Check sheet for the modelled part. Datum: model origin and axes. Units: mm. Face numbers are marked on the shaded views. A direction names the side the tool comes from. Round coordinates to 2 decimals unless told otherwise and drop trailing zeros. Write each loop counter-clockwise with the first axis right and the second up, starting at its lowest first coordinate (ties: lowest second). Pieces come first, ordered by that corner, then holes. Notation, with made-up numbers: (6.25, -26.5) -> (25.25, -26.5) arc R35 ccw to (25.25, 10.5) -> close; hole circle Ø1 at (25.25, -3). An arc over 180 degrees is marked (long way). One line per item, written item: value.
Autodesk Inventor part; units mm, degrees
ref_plane "YZ Plane" through (0, 0, 0) normal (1, 0, 0) x (0, 1, 0)
ref_plane "XZ Plane" through (0, 0, 0) normal (0, 1, 0) x (-1, 0, 0)
ref_plane "XY Plane" through (0, 0, 0) normal (0, 0, 1) x (1, 0, 0)
sketch "Sketch1" plane through (0, 0, 0) normal (0, 0, 1) x (1, 0, 0)
  line L0 (0, 0) -> (55, 0)
  line L1 (55, 0) -> (55, 80)
  line L2 (55, 80) -> (0, 80)
  line L3 (0, 80) -> (0, 0)
  dimension "d0" = 55
  dimension "d1" = 80
extrude "Base" add sketch "Sketch1" along normal blind 2
sketch "Sketch2" plane through (0, 0, 2) normal (0, 0, 1) x (1, 0, 0)
  line L0 (55, 0) -> (55, 80)
  line L1 (0, 80) -> (0, 0)
  line L2 (-2, 0) -> (57, 0)
  line L3 (57, 0) -> (57, 3)
  line L4 (57, 3) -> (-2, 3)
  line L5 (-2, 3) -> (-2, 0)
  dimension "d4" = 3
  dimension "d5" = 2
  dimension "d6" = 2
extrude "Back" add sketch "Sketch2" along normal blind 36.5 and the other way blind 2
sketch "Sketch6" plane through (0, 0, 2) normal (0, 0, 1) x (1, 0, 0)
  line L0 (0, 80) -> (0, 3)
  line L1 (0, 3) -> (55, 3)
  line L2 (55, 3) -> (55, 80)
  line L3 (2, 3) -> (53, 3)
  line L4 (53, 3) -> (53, 38)
  line L5 (53, 38) -> (2, 38)
  line L6 (2, 38) -> (2, 3)
  point P0 (0, 0)
  dimension "d29" = 35
  dimension "d30" = 2
  dimension "d31" = 2
extrude "Box" add sketch "Sketch6" along normal blind 13.5
chamfer "Chamfer3" distance 0.5 angle 45 8 edges at (0, 41.5, 0) (27.5, 80, 0) (55, 41.5, 0) (-1, 3, 0) (-2, 1.5, 0) (27.5, 0, 0) (57, 1.5, 0) (56, 3, 0)
chamfer "Chamfer4" distance 0.5 angle 45 3 edges at (-2, 0, 19.5) (27.5, 0, 38.5) (57, 0, 19.5)
chamfer "Chamfer5" distance 0.5 angle 45 3 edges at (-2, 1.75, 38.5) (27.5, 3, 38.5) (57, 1.75, 38.5)
sketch "Sketch7" plane through (0, 0, 15.5) normal (0, 0, 1) x (1, 0, 0)
  line L0 (53, 3) -> (2, 3)
  line L1 (53, 3) -> (53, 38)
  line L2 (53, 38) -> (2, 38)
  line L3 (2, 38) -> (2, 3)
  line L4 (3.6, 3) -> (51.4, 3)
  line L5 (51.4, 3) -> (51.4, 18.9)
  line L6 (51.4, 18.9) -> (3.6, 18.9)
  line L7 (3.6, 18.9) -> (3.6, 3)
  line L8 (51.4, 36.4) -> (3.6, 36.4)
  line L9 (3.6, 36.4) -> (3.6, 20.5)
  line L10 (3.6, 20.5) -> (51.4, 20.5)
  line L11 (51.4, 20.5) -> (51.4, 36.4)
  point P0 (0, 0)
  dimension "d44" = 1.6
  dimension "d45" = 1.6
  dimension "d46" = 1.6
  dimension "d47" = 1.6
  dimension "d48" = 1.6
  dimension "d49" = 1.6
  dimension "d50" = 15.9
  dimension "d51" = 15.9
extrude "Box inside" cut sketch "Sketch7" against normal blind 13.5 contours L0 L7 L6 L5 | L11 L10 L9 L8
sketch "Sketch8" plane through (0, 0, 2) normal (0, 0, 1) x (1, 0, 0)
  line L0 (55, 3) -> (55, 80)
  line L1 (55, 80) -> (0, 80)
  line L2 (0, 80) -> (0, 3)
  line L3 (22.5, 80) -> (32.5, 80)
  line L4 (32.5, 80) -> (32.5, 77.1)
  line L5 (32.5, 77.1) -> (22.5, 77.1)
  line L6 (22.5, 77.1) -> (22.5, 80)
  point P0 (0, 0)
  dimension "d63" = 22.5
  dimension "d64" = 22.5
  dimension "d65" = 10
  dimension "d66" = 2.9
extrude "Extrusion8" add sketch "Sketch8" along normal blind 1.5
chamfer "Chamfer9" distance 1.5 angle 45 1 edges at (27.5, 77.1, 3.5)
chamfer "Chamfer10" distance 1.4 angle 45 1 edges at (27.5, 80, 3.5)
sketch "Sketch9" plane through (0, 0, 0) normal (0, 0, -1) x (-1, 0, 0)
  line L0 (-58.372, 83.6354) -> (-49.5119, 83.6354)
  line L1 (-49.5119, 83.6354) -> (-49.5119, 74.6368)
  line L2 (-49.5119, 74.6368) -> (-58.372, 74.6368)
  line L3 (-58.372, 74.6368) -> (-58.372, 83.6354)
  line L4 (-5.9034, 83.6354) -> (3.372, 83.6354)
  line L5 (3.372, 83.6354) -> (3.372, 74.6368)
  line L6 (3.372, 74.6368) -> (-5.9034, 74.6368)
  line L7 (-5.9034, 74.6368) -> (-5.9034, 83.6354)
  line L8 (-4.6575, 9.1548) -> (5.0333, 9.1548)
  line L9 (5.0333, 9.1548) -> (5.0333, -3.8585)
  line L10 (5.0333, -3.8585) -> (-4.6575, -3.8585)
  line L11 (-4.6575, -3.8585) -> (-4.6575, 9.1548)
  line L12 (-50.8963, 9.1548) -> (-59.7564, 9.1548)
  line L13 (-59.7564, 9.1548) -> (-59.7564, -3.8585)
  line L14 (-59.7564, -3.8585) -> (-50.8963, -3.8585)
  line L15 (-50.8963, -3.8585) -> (-50.8963, 9.1548)
  point P0 (0, 0)
extrude "printing support" add sketch "Sketch9" against normal blind 0.2
equation "\"d31\" = d30"
equation "\"d45\" = d44"
equation "\"d46\" = d45"
equation "\"d47\" = d46"
equation "\"d48\" = d44"
equation "\"d49\" = d44"
equation "\"d64\" = d63"
properties part number "BOTTOM"
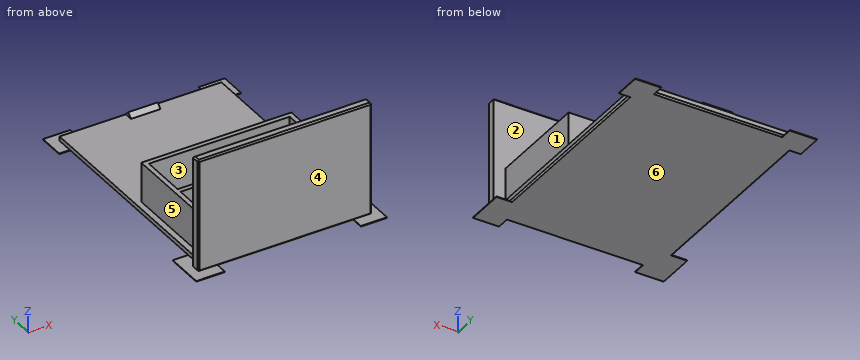
Item 1: Sectioned sample at C-C (y = 35). Enter the section's corners in (x, z), then the cut area to 3 significant figures.
Result set:
outline: (0, 0.5) -> (0.5, 0) -> (54.5, 0) -> (55, 0.5) -> (55, 2) -> (53, 2) -> (53, 15.5) -> (51.4, 15.5) -> (51.4, 2) -> (3.6, 2) -> (3.6, 15.5) -> (2, 15.5) -> (2, 2) -> (0, 2) -> close
area: 153 mm^2
Item 2: Sectioned sample at D-D (z = 18). Enter the section's corners in (x, y), then the cut area to 3 significant figures.
Result set:
outline: (-2, 0.5) -> (-1.5, 0) -> (56.5, 0) -> (57, 0.5) -> (57, 3) -> (-2, 3) -> close
area: 177 mm^2
Item 3: Material ranges on line 1 along X through (y, z) = (33, 7); line 2 along Y through (x, z) = (48, 2.5); line 3 along Z through (x, y) = (43, 40), recorded low to high.
Result set:
line 1: 2 to 3.6, 51.4 to 53
line 2: 0 to 3, 18.9 to 20.5, 36.4 to 38
line 3: 0 to 2
Item 4: Depth check by flat-ended pin: pin 1 (11 mm diameter, centred on x = 33, z = 7.5, fed in from +Y); pin 2 (12 mm diameter, centred on x = 21.5, z = 32.5, fed in from -Y); pin 3 (3 mm diameter, centred on y = 1.5, z = 24.5, fed in from -X). Enter the tip coordinate at first touch or a pass-through.
Result set:
pin 1: y = 80
pin 2: y = 0
pin 3: x = -2
Item 5: Release check for a two-part mould opening along Y. For the marked faces 1, 2, 3 and 4 record: pulls with the +Y half, pulls with the -Y half, needs draft (parallel to the pull), parting line crosses it, or undercut.
Result set:
face 1: needs draft
face 2: undercut
face 3: undercut
face 4: pulls with the -Y half
Item 6: Sectioned sample at A-A (z = 10). Enter the section's corners in (x, y), then the cut area to 3 significant figures.
Result set:
outline: (-2, 0.5) -> (-1.5, 0) -> (56.5, 0) -> (57, 0.5) -> (57, 3) -> (53, 3) -> (53, 38) -> (2, 38) -> (2, 3) -> (-2, 3) -> close; hole (3.6, 3) -> (51.4, 3) -> (51.4, 18.9) -> (3.6, 18.9) -> close; hole (3.6, 20.5) -> (51.4, 20.5) -> (51.4, 36.4) -> (3.6, 36.4) -> close
area: 442 mm^2
Item 7: Tool access check on the marked faces 5 and 6. Record the directions out of +Z, -Z, +X, -X, +Y, -Y that give a thin tool (end or side, any length) a straight path to the whole face; none if there is none.
Result set:
face 5: +Z, -X, +Y
face 6: -Z, +X, -X, +Y, -Y
